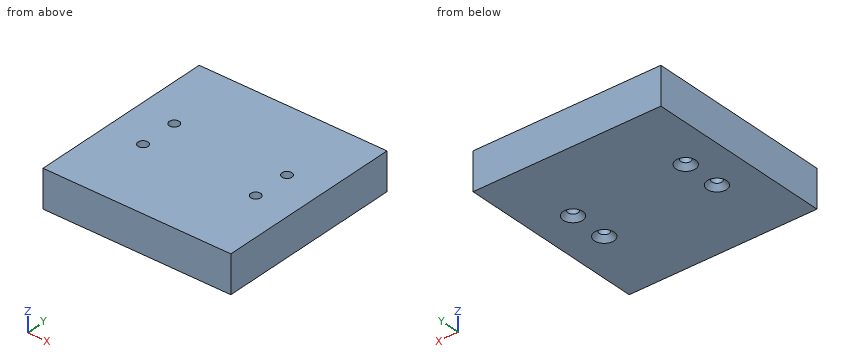
from build123d import *

# Parameters (mm, degrees)
SKETCH1_W                                       = 100
SKETCH1_H                                       = 100
BOSS_EXTRUDE1_DEPTH                             = 20
CSK_FOR_M5_FLAT_HEAD_MACHINE_SCREW1_D           = 5.3
CSK_FOR_M5_FLAT_HEAD_MACHINE_SCREW1_CSINK_D     = 10.4
CSK_FOR_M5_FLAT_HEAD_MACHINE_SCREW1_CSINK_ANGLE = 90


with BuildPart() as part:
    # Sketch1 → Boss-Extrude1 (new body)
    with BuildSketch(Plane.XY):
        Rectangle(SKETCH1_W, SKETCH1_H)
    extrude(amount=BOSS_EXTRUDE1_DEPTH)

    # CSK for M5 Flat Head Machine Screw1 (through all)
    with Locations(Plane(origin=(0, 0, 0), x_dir=(-1, 0, 0), z_dir=(0, 0, -1))):
        with Locations((-30, 10), (30, 10), (30, -10), (-30, -10)):
            CounterSinkHole(CSK_FOR_M5_FLAT_HEAD_MACHINE_SCREW1_D / 2, CSK_FOR_M5_FLAT_HEAD_MACHINE_SCREW1_CSINK_D / 2, counter_sink_angle=CSK_FOR_M5_FLAT_HEAD_MACHINE_SCREW1_CSINK_ANGLE)


solid = part.part
Read the model definition and answer for the solid it produces. Units are mm, in the model's axes. Give positions to 0.01 mm unless a question says otherwise; leave off trailing zeros. Loops run counter-clockwise (first coordinate to the right, second up) from the corner with the lowest first, then second, coordinate; pieces in that order, holes last. Notation, with made-up numbers: (68.25, -16.75) -> (123.25, -16.75) arc R7 cw to (123.25, -7.75) -> close; hole circle Ø8 at (36, -31.75). An arc over 180 degrees is marked (long way). Answer as CSV lines item,"result".
Item 1: Consider line 1 (X direction, y = -10, z = 9); line 2 (Y direction, x = -30, z = 12.75); line 3 (X direction, y = -9, z = 13.75). Determine where each line is inside the solid, lowest interval first. Write a range as [from, to].
Returned:
line 1,"x = [-50, -32.65], [-27.35, 27.35], [32.65, 50]"
line 2,"y = [-50, -12.65], [-7.35, 7.35], [12.65, 50]"
line 3,"x = [-50, -32.45], [-27.55, 27.55], [32.45, 50]"
Item 2: Each of these flat-tipped pins is pushed along its axis until it touches: pin 1 (4 mm diameter, centred on x = -30, y = 10, fed in from -Z); pin 2 (8.5 mm diameter, centred on x = 30, y = -10, fed in from -Z). Where does it stop, or does it pass through?
Returned:
pin 1,"passes through"
pin 2,"stops at z = 0.95"
Item 3: Find section B-B on y = 10. Give the vertices of the cut face in (x, z), plus the area to 4 significant figures.
Returned:
outline,"(-50, 0) -> (-35.2, 0) -> (-32.65, 2.55) -> (-32.65, 20) -> (-50, 20) -> close; (-27.35, 2.55) -> (-24.8, 0) -> (24.8, 0) -> (27.35, 2.55) -> (27.35, 20) -> (-27.35, 20) -> close; (32.65, 2.55) -> (35.2, 0) -> (50, 0) -> (50, 20) -> (32.65, 20) -> close"
area,"1,775 mm²"
Item 4: Find section A-A on x = -30. Give the vertices of the cut face in (y, z).
Returned:
outline,"(-50, 0) -> (-15.2, 0) -> (-12.65, 2.55) -> (-12.65, 20) -> (-50, 20) -> close; (-7.35, 2.55) -> (-4.8, 0) -> (4.8, 0) -> (7.35, 2.55) -> (7.35, 20) -> (-7.35, 20) -> close; (12.65, 2.55) -> (15.2, 0) -> (50, 0) -> (50, 20) -> (12.65, 20) -> close"
